The model under review builds one solid part; all positions refer to its coordinate system, in mm. Face numbers are marked on the shaded views. A direction names the side the tool comes from. Give positions to 0.01 mm unless a question says otherwise; leave off trailing zeros. Order: outer loops, then holes, each group sorted by start corner. A loop starts at its lowest first (then second) coordinate and runs counter-clockwise, first axis right, second up. Notation, with made-up numbers: (57.25, 50.25) -> (112.25, 50.25) arc R36 ccw to (112.25, 87.25) -> close; hole circle Ø2 at (18.25, 53). An arc over 180 degrees is marked (long way). Answer as a JSON object with one key per item and string values. Group by question number.
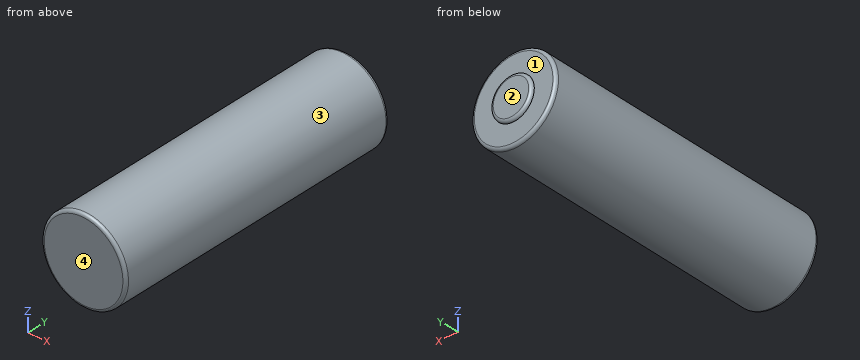
from build123d import *

# Parameters (mm, degrees)
SKETCH1_R           = 7.15
BOSS_EXTRUDE1_DEPTH = 24.5635
SKETCH2_R           = 3.5
BOSS_EXTRUDE2_DEPTH = 0.5
FILLET1_R           = 0.5


with BuildPart() as part:
    # Sketch1 → Boss-Extrude1 (new, symmetric)
    with BuildSketch(Plane(origin=(0, 0, 0), x_dir=(1, 0, 0), z_dir=(0, 1, 0))):
        with Locations(Location((0, 0, 0), (0, 0, 270))):
            Circle(SKETCH1_R)
    extrude(amount=BOSS_EXTRUDE1_DEPTH, both=True)

    # Sketch2 → Boss-Extrude2 (add)
    with BuildSketch(Plane(origin=(0, 24.5635, 0), x_dir=(1, 0, 0), z_dir=(0, 1, 0))):
        with Locations(Location((0, 0, 0), (0, 0, 270))):
            Circle(SKETCH2_R)
    extrude(amount=BOSS_EXTRUDE2_DEPTH)

    # Fillet1
    fillet1_edges = [part.edges().sort_by_distance(p)[0] for p in [
        (0, -24.5635, -7.15),
        (0, 24.5635, -7.15),
        (0, 25.0635, -3.5),
    ]]
    fillet(fillet1_edges, radius=FILLET1_R - 0.0001)  # a hair under: the kernel refuses the full size


solid = part.part
1. Take a section at A-A on y = -19.5. Give the boundary of the cut face in (x, z), plus the area to 3 significant figures.
2. Draft analysis for pull direction X (two halves, no side actions). For the marked faces 3 and 4, state which applies: pulls with the +X half, pulls with the -X half, needs draft (parallel to the pull), parting line crosses it, or undercut.
3. For pin 1 (1 mm diameter, centred on y = -7.5, z = 1.5, fed in from +X); pin 2 (8 mm diameter, centred on x = 5, y = 10.5, fed in from +Z), all flat-tipped, find the tip position at first contact; note any pin that passes through.
4. For probe 1 along Y at (x, z) = (-5.75, -2.25); probe 2 along X at (y, z) = (-20, -0.25), list the stretches that pass through material, from the lowest coordinate up. Write a range as [from, to].
5. Machinability: for the marked faces 1 and 2, which of the approach directions +Z, -Z, +X, -X, +Y, -Y give a long, thin tool a straight path to every point of the face, cutting with its end or side? Answer none if there is none.
Checks:
{
 "1": {"outline": "circle Ø14.3 at (0, 0)", "area": "161 mm2"},
 "2": {"face 3": "parting line crosses it", "face 4": "needs draft"},
 "3": {"pin 1": "stops at x = 7.08", "pin 2": "stops at z = 7.08"},
 "4": {"probe 1": "y = [-24.56, 24.56]", "probe 2": "x = [-7.15, 7.15]"},
 "5": {"face 1": "+Y", "face 2": "+Z, -Z, +X, -X, +Y"}
}
